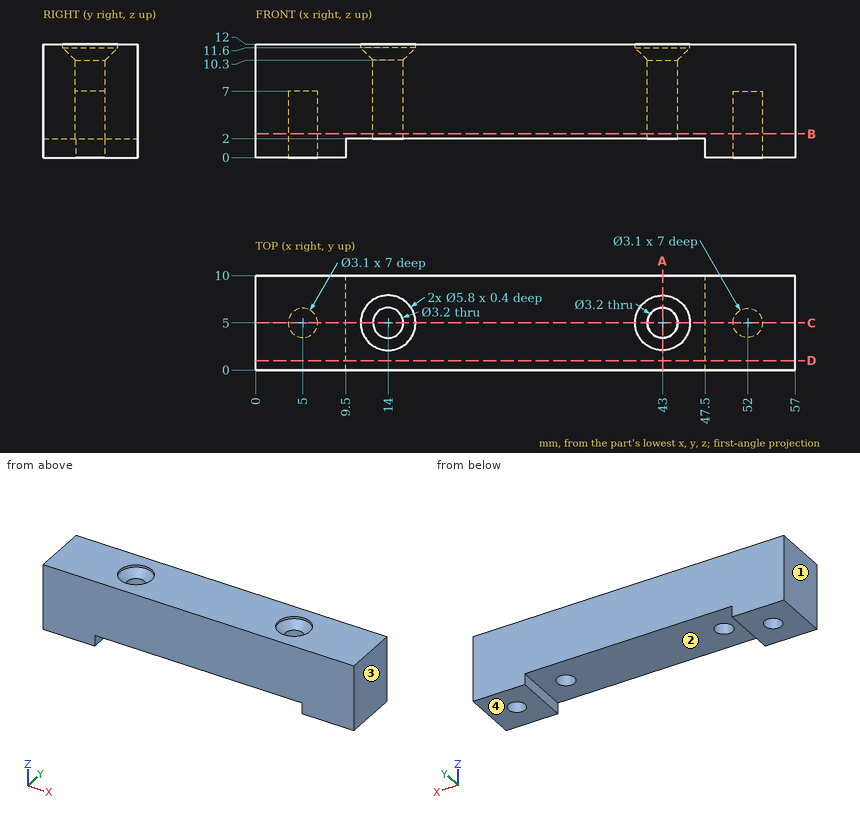
Could you check a few things on this drawing? It's one solid part, dimensions in mm from its lowest x, y, z. Coordinates: 2 decimals unless noted, no trailing zeros. Order: outer loops, then holes, each group sorted by start corner. A loop starts at its lowest first (then second) coordinate and runs counter-clockwise, first axis right, second up.
1. If we section it at A-A (x = 43): Please give me the cut outline in (y, z).
2. If we section it at D-D (y = 1): Please give me the cut outline in (x, z), then the cut area to 3 significant figures.
3. I need wall thicknesses on line 1 (X direction, y = 5, z = 11.9); line 2 (X direction, y = 5, z = 8.75); line 3 (Y direction, x = 43, z = 11.8). Which ranges of each line are inside material? Lowest first, please.
4. I'm going to push flat-ended pins straight in: pin 1 (5 mm diameter, centred on x = 14, y = 5, fed in from -Z); pin 2 (1.5 mm diameter, centred on x = 52, y = 5.5, fed in from -Z); pin 3 (2 mm diameter, centred on x = 18, z = 6.5, fed in from -Y); pin 4 (2.5 mm diameter, centred on x = 43, y = 5, fed in from -Z). Where does each tip first touch, or does it pass through?
5. Thinking about a two-plate mould opening in X: for the marked faces 1, 2, 3 and 4, which applies, +X half, -X half, draft (parallel to the pull), parting line (faces both ways), or undercut?
6. If we section it at B-B (z = 2.5): Please give me the cut outline in (x, y), then the cut area to 3 significant figures.
7. If we section it at C-C (y = 5): Give the number of separate pieces and of enclosed holes in the cut face, then the cut area to 3 significant figures.
Entries:
1. outline: (0, 2) - (3.4, 2) - (3.4, 10.3) - (2.1, 11.6) - (2.1, 12) - (0, 12) - close; (6.6, 2) - (10, 2) - (10, 12) - (7.9, 12) - (7.9, 11.6) - (6.6, 10.3) - close
2. outline: (0, 0) - (9.5, 0) - (9.5, 2) - (47.5, 2) - (47.5, 0) - (57, 0) - (57, 12) - (0, 12) - close
2. area: 608 mm2
3. line 1: x = 0 to 11.1, 16.9 to 40.1, 45.9 to 57
3. line 2: x = 0 to 12.4, 15.6 to 41.4, 44.6 to 57
3. line 3: y = 0 to 2.1, 7.9 to 10
4. pin 1: stops at z = 2
4. pin 2: stops at z = 7
4. pin 3: stops at y = 0
4. pin 4: passes through
5. face 1: -X half
5. face 2: undercut
5. face 3: +X half
5. face 4: draft
6. outline: (0, 0) - (57, 0) - (57, 10) - (0, 10) - close; hole circle Ø3.1 at (5, 5); hole circle Ø3.2 at (14, 5); hole circle Ø3.2 at (43, 5); hole circle Ø3.1 at (52, 5)
6. area: 539 mm2
7. separate pieces: 3
7. enclosed holes: 0
7. area: 495 mm2
